```python
from build123d import *

# Parameters (mm, degrees)
SKETCH2_R                  = 3.175
BOSS_EXTRUDE1_DEPTH        = 4.7625
BOSS_EXTRUDE2_START        = 12.7
BOSS_EXTRUDE2_DEPTH        = 12.7
SKETCH12_W                 = 6.477
SKETCH12_H                 = 13.919150617
SKETCH12_H_2               = 7.9375
CUT_EXTRUDE1_DEPTH         = 24.13
SKETCH12_3_W               = 6.477
SKETCH12_3_H               = 4.7625
CUT_EXTRUDE2_DEPTH         = 19.05
TAP_DRILL_FOR_10_32_TAP1_D = 4.0386
F_1_4_CLEARANCE_HOLE1_D    = 6.5278


with BuildPart() as part:
    # Sketch2 → Boss-Extrude1 (new body)
    with BuildSketch(Plane.XY):
        with BuildLine():
            Line((-67.986186343, -228.533359856), (-69.686856366, -224.252380141))
            Line((-69.686856366, -224.252380141), (-61.0470258, -221.260552334))
            Line((-61.0470258, -221.260552334), (-48.895, -221.260552334))
            Line((-48.895, -221.260552334), (-48.895, -203.133359856))
            ThreePointArc((-48.895, -203.133359856), (-45.175256121, -194.153103735), (-36.195, -190.433359856))
            Line((-36.195, -190.433359856), (25.4, -190.433359856))
            Line((25.4, -190.433359856), (25.4, -228.533359856))
            Line((25.4, -228.533359856), (-67.986186343, -228.533359856))
        make_face()
        with Locations(Location((-36.195, -203.133359856, 0), (0, 0, 180))):
            Circle(SKETCH2_R, mode=Mode.SUBTRACT)
    extrude(amount=BOSS_EXTRUDE1_DEPTH)

    # Sketch11 → Boss-Extrude2 (add)
    with BuildSketch(Plane(origin=(0, 0, 0), x_dir=(-1, 0, 0), z_dir=(0, 0, -1)).offset(BOSS_EXTRUDE2_START)):
        with BuildLine():
            Line((25.4, -190.433359856), (25.4, -228.533359856))
            Line((25.4, -228.533359856), (67.986186343, -228.533359856))
            Line((67.986186343, -228.533359856), (69.686856366, -224.252380141))
            Line((69.686856366, -224.252380141), (61.0470258, -221.260552334))
            Line((61.0470258, -221.260552334), (48.895, -221.260552334))
            Line((48.895, -221.260552334), (48.895, -203.133359856))
            ThreePointArc((48.895, -203.133359856), (45.175256121, -194.153103735), (36.195, -190.433359856))
            Line((36.195, -190.433359856), (25.4, -190.433359856))
        make_face()
    extrude(amount=-BOSS_EXTRUDE2_DEPTH)

    # Sketch12 → Cut-Extrude1 (cut)
    with BuildSketch(Plane.ZY.offset(48.895)):
        with Locations((-3.2385, -210.092935165)):
            Rectangle(SKETCH12_W, SKETCH12_H)
        with Locations((-3.2385, -199.164609856)):
            Rectangle(SKETCH12_W, SKETCH12_H_2)
    extrude(amount=-CUT_EXTRUDE1_DEPTH, mode=Mode.SUBTRACT)

    # Sketch12_3 → Cut-Extrude2 (cut)
    with BuildSketch(Plane.ZY.offset(48.895)):
        with Locations((-3.2385, -192.814609856)):
            Rectangle(SKETCH12_3_W, SKETCH12_3_H)
    extrude(amount=-CUT_EXTRUDE2_DEPTH, mode=Mode.SUBTRACT)

    # Tap Drill for _10-32 Tap1 (through all)
    with Locations(Plane.XY.offset(-6.477)):
        with Locations((-36.195, -203.133359856)):
            Hole(TAP_DRILL_FOR_10_32_TAP1_D / 2)

    # 1_4 Clearance Hole1 (through all)
    with Locations(Plane.XY.offset(4.7625)):
        with Locations((-10.8204, -198.370859856), (-10.8204, -220.595859856), (10.8204, -220.595859856), (10.8204, -198.370859856)):
            Hole(F_1_4_CLEARANCE_HOLE1_D / 2)


solid = part.part
```
Source: CAD feature listing. Evaluate the final solid. Frame: model axes, mm. A direction names the side the tool comes from. Round coordinates to 2 decimals unless told otherwise and drop trailing zeros. Loops run counter-clockwise (first coordinate to the right, second up) from the corner with the lowest first, then second, coordinate; pieces in that order, holes last. Notation, with made-up numbers: M 61.25,36 L 77.25,36 A14 ccw 77.25,57 Z; hole C 55.25,45.25 d3. An arc over 180 degrees is marked long. Use a Markdown table: item, result. Add a question column.
1. Ray query, line 1 along X through (y, z) = (-199.5, 1.25); line 2 along Z through (x, y) = (-27, -203.5); line 3 along X through (y, z) = (-192.5, -4.75) (3 decimals). Return the intervals inside material, ascending. Write a range as [from, to].
2. Cut plane A-A, the plane x = -31.5. Output: boundary loops of the cut face in (y, z).
3. Contact query for flat-ended pins moving along their axis: pin 1 (5 mm diameter, centred on y = -216.5, z = -0.5, fed in from -X) (3 decimals); pin 2 (1.9 mm diameter, centred on x = -31.5, z = -2.5, fed in from +Y); pin 3 (3.5 mm diameter, centred on x = -36.2, y = -203.13, fed in from -Z); pin 4 (1.5 mm diameter, centred on y = -210, z = -7, fed in from +X). Output: stop coordinate, or through.
4. Cut plane C-C, the plane z = -10. Output: boundary loops of the cut face in (x, y) (3 decimals).
5. Cut plane B-B, the plane y = -213. Output: boundary loops of the cut face in (x, z) (1 decimal), and give its area (3 significant figures).
6. Cut plane D-D, the plane y = -219.5. Output: boundary loops of the cut face in (x, z) (1 decimal), and give its area (3 significant figures).
7. Set-up query: faces 1 (the cylindrical face through (-35.78, -206.28, 2.35)), 2 (the flat face through (-37, -207, -6.477)), 3 (the flat face through (-29.845, -193, -3)), 4 (the flat face through (-48.895, -214, -8)). Return all of +Z, -Z, +X, -X, +Y, -Y with unobstructed straight access to the full face (end or side cutting, diameter ignored); none if empty.
8. Pull-direction query (X, two-part tool) for faces 5 (the cylindrical face through (9.314, -201.267, 2.348)), 6 (the flat face through (25.4, -209, 2)), 7 (the flat face through (-11, -209, 4.762)); classes: +X half, -X half, draft (parallel to the pull), parting line (faces both ways), or undercut.
Solution:
| question | item | result |
|---|---|---|
| 1 | line 1 | x = [-48.36, -13.88], [-7.76, 7.76], [13.88, 25.4] |
| 1 | line 2 | z = [-12.7, -6.48], [0, 4.76] |
| 1 | line 3 | x = [-29.845, -25.4] |
| 2 | outline | M -228.53,-12.7 L -190.43,-12.7 L -190.43,-6.48 L -217.05,-6.48 L -217.05,0 L -190.43,0 L -190.43,4.76 L -228.53,4.76 Z |
| 3 | pin 1 | stops at x = -48.895 |
| 3 | pin 2 | stops at y = -217.05 |
| 3 | pin 3 | passes through |
| 3 | pin 4 | stops at x = -25.4 |
| 4 | outline | M -69.687,-224.252 L -67.986,-228.533 L -25.4,-228.533 L -25.4,-190.433 L -36.195,-190.433 A12.7 ccw -48.895,-203.133 L -48.895,-221.261 L -61.047,-221.261 Z; hole C -36.195,-203.133 d4.039 |
| 5 | outline | M -48.9,-12.7 L -25.4,-12.7 L -25.4,-6.5 L -48.9,-6.5 Z; M -48.9,0 L 25.4,0 L 25.4,4.8 L -48.9,4.8 Z |
| 5 | area | 500 mm2 |
| 6 | outline | M -48.9,-12.7 L -25.4,-12.7 L -25.4,0 L -13.9,0 L -13.9,4.8 L -48.9,4.8 Z; M -7.7,0 L 7.7,0 L 7.7,4.8 L -7.7,4.8 Z; M 13.9,0 L 25.4,0 L 25.4,4.8 L 13.9,4.8 Z |
| 6 | area | 594 mm2 |
| 7 | face 1 | +Z |
| 7 | face 2 | -X |
| 7 | face 3 | -X, +Y |
| 7 | face 4 | +Z, -Z, -X, +Y |
| 8 | face 5 | undercut |
| 8 | face 6 | +X half |
| 8 | face 7 | draft |
